Can you work these out from the model? Positions are in its coordinate system, mm. Give positions to 0.01 mm unless a question says otherwise; leave off trailing zeros. Order: outer loops, then holes, each group sorted by start corner. A loop starts at its lowest first (then second) coordinate and runs counter-clockwise, first axis right, second up. Notation, with made-up numbers: (-18.5, 88) - (24.5, 88) arc R11 cw to (24.5, 104) - close; hole circle Ø4 at (-8, 34). An arc over 180 degrees is marked (long way). Use one line per item in the form item = value. Start each with the question number.
1) For pin 1 (3 mm diameter, centred on x = 4.445, y = -20.32, fed in from +Z), with a flat end and sliding along its axis, tell me the tip position at first contact or that it passes through.
2) Suppose I cut it at A-A, the plane y = -83.82. Write out the boundary of the cut face in (x, z).
3) Suppose I cut it at C-C, the plane z = 1.05. Write out the boundary of the cut face in (x, y) (3 decimals), and give its area (3 significant figures).
4) Please list where these lines run through material, in increasing order: probe 1 along Y at (x, z) = (4.25, 1); probe 2 along X at (y, z) = (-83.82, 0.45); probe 3 along Y at (x, z) = (8.5, 0.1).
5) Suppose I cut it at B-B, the plane x = 10.5. Write out the boundary of the cut face in (y, z).
```python
from build123d import *

# Parameters (mm, degrees)
SKETCH1_W          = 19.05
SKETCH1_H          = 95.25
EXTRUDE1_DEPTH     = 1.6002
SKETCH2_R          = 1.8034
CUT_EXTRUDE1_DEPTH = 1.6002
SKETCH3_R          = 1.778
CUT_EXTRUDE2_DEPTH = 2.54


with BuildPart() as part:
    # Sketch1 → Extrude1 (new body)
    with BuildSketch(Plane.XY):
        with Locations((9.525, -47.625)):
            Rectangle(SKETCH1_W, SKETCH1_H)
    extrude(amount=EXTRUDE1_DEPTH)

    # Sketch2 → Cut-Extrude1 (cut)
    with BuildSketch(Plane.XY.offset(1.6002)):
        with Locations((9.525, -6.35)):
            Circle(SKETCH2_R)
    extrude(amount=-CUT_EXTRUDE1_DEPTH, mode=Mode.SUBTRACT)

    # Sketch3 → Cut-Extrude2 (cut)
    with BuildSketch(Plane.XY.offset(1.6002)):
        with Locations((4.445, -20.32)):
            Circle(SKETCH3_R)
        with Locations((4.445, -83.82)):
            Circle(SKETCH3_R)
    extrude(amount=-CUT_EXTRUDE2_DEPTH, mode=Mode.SUBTRACT)


solid = part.part
```
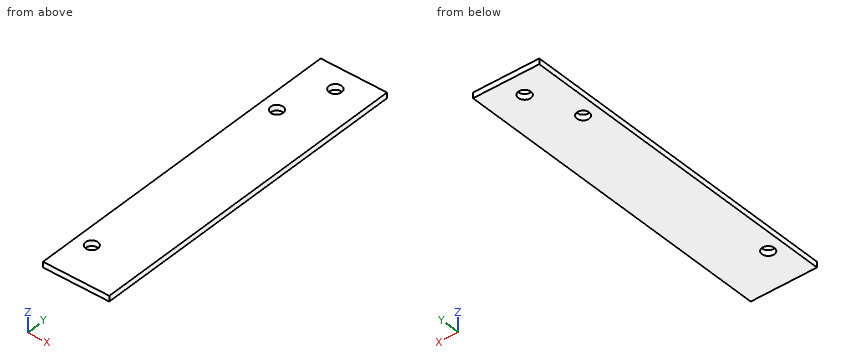
Result sheet:
q1.pin_1 = through
q2.outline = (0, 0) - (2.67, 0) - (2.67, 1.6) - (0, 1.6) - close; (6.22, 0) - (19.05, 0) - (19.05, 1.6) - (6.22, 1.6) - close
q3.outline = (0, -95.25) - (19.05, -95.25) - (19.05, 0) - (0, 0) - close; hole circle Ø3.556 at (4.445, -83.82); hole circle Ø3.556 at (4.445, -20.32); hole circle Ø3.607 at (9.525, -6.35)
q3.area = 1,780 mm²
q4.probe_1 = -95.25 to -85.59, -82.05 to -22.09, -18.55 to 0
q4.probe_2 = 0 to 2.67, 6.22 to 19.05
q4.probe_3 = -95.25 to -7.83, -4.87 to 0
q5.outline = (-95.25, 0) - (-7.87, 0) - (-7.87, 1.6) - (-95.25, 1.6) - close; (-4.83, 0) - (0, 0) - (0, 1.6) - (-4.83, 1.6) - close
